Autodesk Fusion 360 part; units mm, degrees
sketch "Skizze1" plane through (0, 0, 0) normal (1, 0, 0) x (0, 0, -1)
  line L0 (21, 21) -> (-21, 21)
  line L1 (-21, 21) -> (-21, -21)
  line L2 (-21, -21) -> (21, -21)
  line L3 (21, -21) -> (21, 21)
  line L4 (21, 21) -> (-21, -21) construction
  line L5 (-21, 21) -> (21, -21) construction
  line L6 (15.5, -15.5) -> (-15.5, -15.5)
  line L7 (-15.5, -15.5) -> (-15.5, 15.5)
  line L8 (-15.5, 15.5) -> (15.5, 15.5)
  line L9 (15.5, 15.5) -> (15.5, -15.5)
  line L10 (15.5, -15.5) -> (-15.5, 15.5) construction
  line L11 (-15.5, -15.5) -> (15.5, 15.5) construction
  circle A0 centre (15.5, -15.5) radius 1.5
  circle A1 centre (-15.5, -15.5) radius 1.5
  circle A2 centre (-15.5, 15.5) radius 1.5
  circle A3 centre (15.5, 15.5) radius 1.5
  circle A4 centre (0, 0) radius 11
  circle A5 centre (0, 0) radius 2.5
  line L12 (0, 0) -> (2, 0)
  line L13 (2, 0) -> (2, 1.5)
  line L14 (2, 0) -> (2, -1.5)
  dimension "d1" = 42
  dimension "d2" = 42
  dimension "d5" = 31
  dimension "d6" = 31
  dimension "d7" = 3
  dimension "d8" = 3
  dimension "d9" = 3
  dimension "d10" = 3
  dimension "d13" = 22
  dimension "d16" = 5
  dimension "d20" = 2
extrude "Extrusion1" add sketch "Skizze1" against normal blind 37.5 contours L0 L1 L2 L3 | L6 L7 A1 | L6 L7 L8 L9 A0 A1 A2 A3 | L6 L7 A1 | L6 L9 A0 | L6 L9 A0 | L7 L8 A2 | L7 L8 A2 | L8 L9 A3 | L8 L9 A3 | A4 | A5 L13 L14 | A5 L13 L14
extrude "Extrusion2" cut sketch "Skizze1" against normal blind 4 contours L6 L7 A1 | L6 L7 A1 | L6 L9 A0 | L6 L9 A0 | L7 L8 A2 | L7 L8 A2 | L8 L9 A3 | L8 L9 A3
extrude "Extrusion3" add sketch "Skizze1" along normal blind 2 contours A4 | A5 L13 L14 | A5 L13 L14
extrude "Extrusion4" add sketch "Skizze1" along normal blind 23 contours A5 L13 L14 picked at (2.3264, 0.107)
chamfer "Fase1" distance 3 angle 45 4 edges at (-18.75, 21, 21) (-18.75, 21, -21) (-18.75, -21, -21) (-18.75, -21, 21)
CAD build for the part. Positions are in the model's coordinates, mm. A direction names the side the tool comes from. Round coordinates to 2 decimals unless told otherwise and drop trailing zeros. Loops run counter-clockwise (first coordinate to the right, second up) from the corner with the lowest first, then second, coordinate; pieces in that order, holes last. Notation, with made-up numbers: M 88.25,50.5 L 137.25,50.5 A27 ccw 137.25,73.5 Z; hole C 3,-37 d10. An arc over 180 degrees is marked long. One line per question, with ' | ' between items. Start each with the question number.
Item 1: Wall check: line 1 (Y direction, x = -2.35, z = 15.5); line 2 (Y direction, x = -1, z = -15). Give the ranges that are in metal, low to high.
Item 2: Cut at B-B, the plane z = 0. Write the cut outline in (x, y), plus the area to 3 significant figures.
Item 3: Cut at C-C, the plane y = -15.5. Write the cut outline in (x, z), plus the area to 3 significant figures.
Item 4: Two-plate mould, pull along Z, no slides. Class faces 4 (the cylindrical face through (-1.97, 15.57, -14)), 5 (the flat face through (-18, 0, 21)), 6 (the cylindrical face through (0.99, 10.74, 2.38)), 7 (the flat face through (0, 10, 10)): pulls with the +Z half, pulls with the -Z half, needs draft (parallel to the pull), parting line crosses it, or undercut.
Item 5: Which spindle directions (+Z, -Z, +X, -X, +Y, -Y) get a long thin tool onto all of the face, cutting with end or side? Do faces 1 (the cylindrical face through (12.4, 0, -2.5)), 2 (the cylindrical face through (-1.97, -15.43, -14)), 3 (the flat face through (-18, 21, 0)). Say none if no direction does.
Item 6: Cut at A-A, the plane x = -1. Write the cut outline in (y, z).
Item 7: Pin check, flat tips, straight feed: pin 1 Ø2.5 at (y, z) = (15.5, 15.5) entering from +X; pin 2 Ø2.5 at (y, z) = (15, -16) entering from +X; pin 3 Ø12 at (y, z) = (-9.5, -4) entering from +X. Stop position of each tip, or through.
Responses:
1) line 1: y = -21 to -17, -14 to 14, 17 to 21 | line 2: y = -21 to -16.91, -14.09 to 14.09, 16.91 to 21
2) outline: M -37.5,-21 L 0,-21 L 0,-11 L 2,-11 L 2,11 L 0,11 L 0,21 L -37.5,21 Z | area: 1,620 mm²
3) outline: M -37.5,-21 L 0,-21 L 0,-17 L -4,-17 L -4,-14 L 0,-14 L 0,14 L -4,14 L -4,17 L 0,17 L 0,21 L -37.5,21 Z | area: 1,550 mm²
4) face 4: undercut | face 5: pulls with the +Z half | face 6: parting line crosses it | face 7: needs draft
5) face 1: -Z, +X | face 2: +X | face 3: +Z, -Z, +X, -X, +Y
6) outline: M -21,-18 L -18,-21 L 18,-21 L 21,-18 L 21,18 L 18,21 L -18,21 L -21,18 Z; hole C -15.5,-15.5 d3; hole C -15.5,15.5 d3; hole C 15.5,-15.5 d3; hole C 15.5,15.5 d3
7) pin 1: stops at x = -4 | pin 2: stops at x = 0 | pin 3: stops at x = 2
